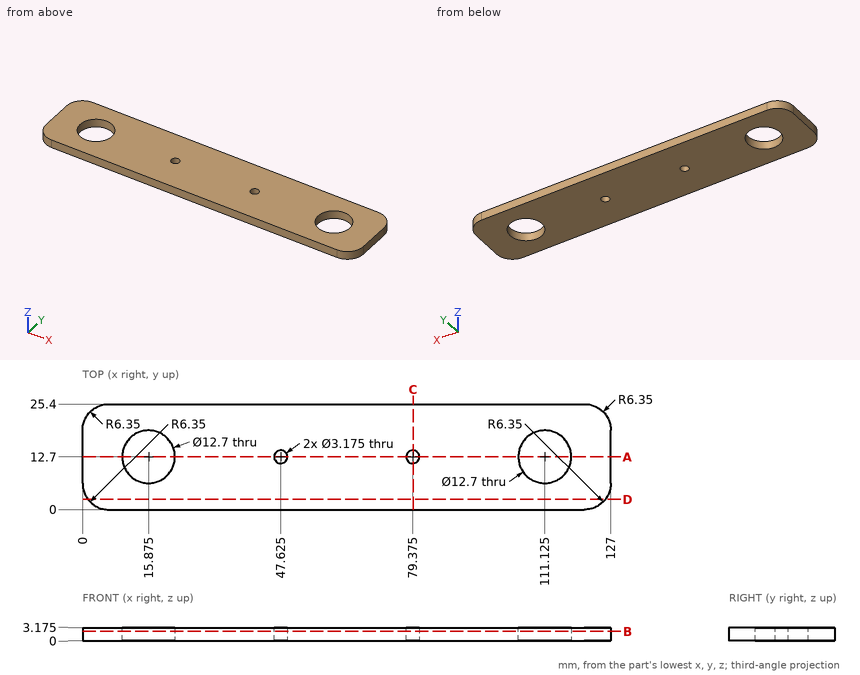
Geometry check sheet. Reference: drawing and pictorial views, mm from the part's lowest x, y, z. Give positions to 0.01 mm unless a question says otherwise; leave off trailing zeros. Loops run counter-clockwise (first coordinate to the right, second up) from the corner with the lowest first, then second, coordinate; pieces in that order, holes last. Notation, with made-up numbers: (-8.5, 49.25) - (44.5, 49.25) arc R35 cw to (44.5, 81.25) - close; hole circle Ø1 at (60.5, -1). An arc over 180 degrees is marked (long way). One line per question, with ' | ' between items. Start each with the question number.
1. Cross-section at C-C, the plane x = 79.5. Enter the section's corners in (y, z) (3 decimals).
2. Cross-section at D-D, the plane y = 2.5. Enter the section's corners in (x, z) (3 decimals).
3. Material ranges on line 1 along Y through (x, z) = (16, 2.75); line 2 along X through (y, z) = (13, 2.1); line 3 along X through (y, z) = (8.25, 2.9), recorded low to high. Write a range as [from, to].
4. Cross-section at A-A, the plane y = 12.7. Enter the section's corners in (x, z) (1 decimal), plus the area to 3 significant figures.
5. Cross-section at B-B, the plane z = 2.3. Give the number of separate pieces and of enclosed holes in the cut face, plus the area to 3 significant figures.
6. Gauge pin test, flat end, axial feed: pin 1 Ø1.9 at (x, y) = (79.375, 12.7) entering from +Z. Record the tip position at first contact, or that the pin passes through.
Check result:
1) outline: (0, 0) - (11.117, 0) - (11.117, 3.175) - (0, 3.175) - close; (14.283, 0) - (25.4, 0) - (25.4, 3.175) - (14.283, 3.175) - close
2) outline: (1.3, 0) - (125.7, 0) - (125.7, 3.175) - (1.3, 3.175) - close
3) line 1: y = [0, 6.35], [19.05, 25.4] | line 2: x = [0, 9.53], [22.22, 46.07], [49.18, 77.82], [80.93, 104.78], [117.47, 127] | line 3: x = [0, 11.35], [20.4, 106.6], [115.65, 127]
4) outline: (0, 0) - (9.5, 0) - (9.5, 3.2) - (0, 3.2) - close; (22.2, 0) - (46, 0) - (46, 3.2) - (22.2, 3.2) - close; (49.2, 0) - (77.8, 0) - (77.8, 3.2) - (49.2, 3.2) - close; (81, 0) - (104.8, 0) - (104.8, 3.2) - (81, 3.2) - close; (117.5, 0) - (127, 0) - (127, 3.2) - (117.5, 3.2) - close | area: 302 mm2
5) separate pieces: 1 | enclosed holes: 4 | area: 2,920 mm2
6) pin 1: passes through
